Can you work these out from the model? Positions are in its coordinate system, mm. A direction names the side the tool comes from. Give positions to 0.01 mm unless a question says otherwise; leave off trailing zeros. Order: outer loops, then holes, each group sorted by start corner. A loop starts at its lowest first (then second) coordinate and runs counter-clockwise, first axis right, second up. Notation, with made-up numbers: M 84,-36.75 L 102,-36.75 A27 ccw 102,-16.75 Z; hole C 80.25,80.5 d1. An arc over 180 degrees is marked long. Use one line per item in the form item = value. Start each with the question number.
1. I want a section at A-A, the plane z = 39. List the corners of the cut face in (x, y) for me.
2. For faces 1 (the face through (28.237, -6.27, 1.521)), 2 (the face through (0, 0, 0)), 3 (the face through (-24.2, 15.43, 38.23)), which set-ups out of +Z, -Z, +X, -X, +Y, -Y let a thin tool reach every point of the face, with its end or its side?
3. We'd pull the mould along X, two halves only. Please class faces 4 (the face through (26.4, 8.7, 48)), 5 (the face through (0, 0, 47.2)), 6 (the face through (28.554, -6.341, 13.915)): +X half, -X half, draft (parallel to the pull), parting line (faces both ways), or undercut.
4. Will these pins go through, and if not, where does the flat tip stop? P1, Ø1, axis at x = -19, z = 6.5, coming from the +Y side; P2, Ø1.5, axis at x = -20, y = -10.5, coming from the +Z side; P3, Ø8, axis at y = 10, z = 13, coming from the -X side.
5. I need wall thicknesses on L1, parallel to Z at x = -16, y = -8; L2, parallel to Y at x = 6.5, z = 5.5; L3, parallel to Z at x = 27, y = 12.5. Which ranges of each line are inside material? Lowest first, please.
```python
from build123d import *


with BuildPart() as f1:
    # F0 (on Right) → F1 (revolve)
    with BuildSketch(Plane.YZ):
        Polygon((0, 0), (28.925, 0), (28.925, 3), (29.25, 3), (29.25, 12.6), (29.2, 12.6), (29.2, 12.8), (29.25, 12.8), (29.25, 15), (28.5, 15), (28.5, 30.5), (29.2, 30.5), (29.2, 32.7), (28.7, 32.7), (28.7, 43.6), (29.85, 43.6), (29.85, 48), (27.5, 48), (26.55, 47.2), (0, 47.2), align=None)
    revolve(axis=Axis((0, 0, 53.454532), (0, 0, 1)))


solid = f1.part
```
Check result:
q1.outline = C 0,0 d57.4
q2.face_1 = -Z
q2.face_2 = -Z, +X, -X, +Y, -Y
q2.face_3 = none
q3.face_4 = draft
q3.face_5 = undercut
q3.face_6 = parting line
q4.P1 = 22.66
q4.P2 = 47.2
q4.P3 = -28.63
q5.L1 = 0 to 47.2
q5.L2 = -28.52 to 28.52
q5.L3 = 43.6 to 48
